Geometry check sheet. Reference: the model listing, model coordinates, mm. Face numbers are marked on the shaded views. Coordinates: 2 decimals unless noted, no trailing zeros. Order: outer loops, then holes, each group sorted by start corner. A loop starts at its lowest first (then second) coordinate and runs counter-clockwise, first axis right, second up. Notation, with made-up numbers: M 14,72 L 69,72 A18 cw 69,82 Z; hole C 24,80.25 d5. An arc over 180 degrees is marked long. One line per item, written item: value. Start each with the question number.
1) Thickness scan on L1, parallel to X at y = 34.1, z = 0; L2, parallel to Y at x = -59.5, z = 21.5; L3, parallel to X at y = 38.7, z = 0. Record the ranges inside material, lowest first. Write a range as from..to.
2) Draft check along X on the marked faces 1, 2 and 3. Enter one of: pulls with the +X half, pulls with the -X half, needs draft (parallel to the pull), parting line crosses it, or undercut.
3) Sectioned sample at B-B, the plane x = 0. Enter the section's corners in (y, z).
4) Go/stop test with flat-tipped pins: P1, Ø12, axis at x = -8, y = 26.5, coming from the -Z side; P2, Ø1.5, axis at x = -5.5, y = 4.5, coming from the +Z side; P3, Ø6, axis at y = 32, z = 0, coming from the +X side. Record where each tip stops, or that it passes through.
5) Sectioned sample at C-C, the plane y = 14. Enter the section's corners in (x, z).
6) Sectioned sample at A-A, the plane z = 0. Enter the section's corners in (x, y).
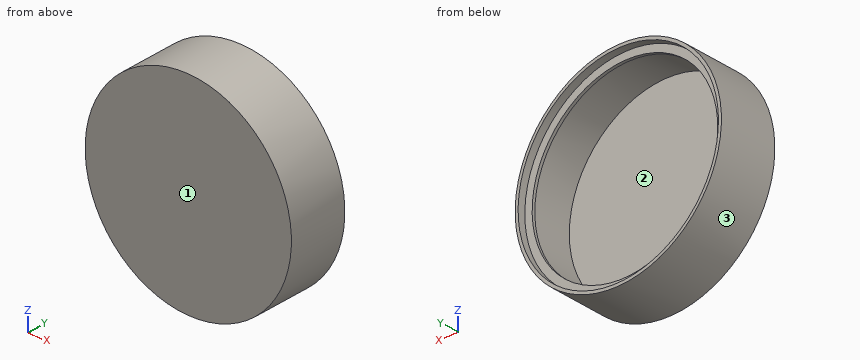
```python
from build123d import *

# Parameters (mm, degrees)
SKETCH2_R           = 70
BOSS_EXTRUDE1_DEPTH = 40
SKETCH4_R           = 63
CUT_EXTRUDE1_DEPTH  = 35
SKETCH5_R           = 68
CUT_EXTRUDE2_DEPTH  = 5
SKETCH6_R           = 65
CUT_EXTRUDE3_DEPTH  = 28


with BuildPart() as part:
    # Sketch2 → Boss-Extrude1 (new body)
    with BuildSketch(Plane(origin=(0, 0, 0), x_dir=(1, 0, 0), z_dir=(0, 1, 0))):
        with Locations(Location((0, 0, 0), (0, 0, 270))):
            Circle(SKETCH2_R)
    extrude(amount=BOSS_EXTRUDE1_DEPTH)

    # Sketch4 → Cut-Extrude1 (cut)
    with BuildSketch(Plane(origin=(0, 40, 0), x_dir=(1, 0, 0), z_dir=(0, 1, 0))):
        with Locations(Location((0, 0, 0), (0, 0, 270))):
            Circle(SKETCH4_R)
    extrude(amount=-CUT_EXTRUDE1_DEPTH, mode=Mode.SUBTRACT)

    # Sketch5 → Cut-Extrude2 (cut)
    with BuildSketch(Plane(origin=(0, 40, 0), x_dir=(1, 0, 0), z_dir=(0, 1, 0))):
        with Locations(Location((0, 0, 0), (0, 0, 270))):
            Circle(SKETCH5_R)
    extrude(amount=-CUT_EXTRUDE2_DEPTH, mode=Mode.SUBTRACT)

    # Sketch6 → Cut-Extrude3 (cut)
    with BuildSketch(Plane(origin=(0, 33, 0), x_dir=(1, 0, 0), z_dir=(0, 1, 0))):
        with Locations(Location((0, 0, 0), (0, 0, 270))):
            Circle(SKETCH6_R)
    extrude(amount=-CUT_EXTRUDE3_DEPTH, mode=Mode.SUBTRACT)


solid = part.part
```
Final values:
1. L1: x = -70..-63, 63..70
1. L2: y = 0..5, 33..35
1. L3: x = -70..-68, 68..70
2. face 1: needs draft
2. face 2: undercut
2. face 3: parting line crosses it
3. outline: M 0,-70 L 40,-70 L 40,-68 L 35,-68 L 35,-63 L 33,-63 L 33,-65 L 5,-65 L 5,65 L 33,65 L 33,63 L 35,63 L 35,68 L 40,68 L 40,70 L 0,70 Z
4. P1: stops at z = -69.97
4. P2: stops at z = 69.84
4. P3: stops at x = 70
5. outline: C 0,0 d140; hole C 0,0 d130
6. outline: M -70,0 L 70,0 L 70,40 L 68,40 L 68,35 L 63,35 L 63,33 L 65,33 L 65,5 L -65,5 L -65,33 L -63,33 L -63,35 L -68,35 L -68,40 L -70,40 Z
